```python
from build123d import *

# Parameters (mm, degrees)
EXTRUDE_1_DEPTH          = 4
SKETCH_3_R               = 4.330127019
SKETCH_3_R_2             = 2
EXTRUDE_2_DEPTH          = 9
SKETCH_4_R               = 1.5
CUT_EXTRUDE_1_DEPTH      = 15
CUT_EXTRUDE_2_DEPTH      = 15.585952146
CUT_EXTRUDE_2_DEPTH_BACK = 15.585952146
SKETCH_5_R               = 1.5


with BuildPart() as part:
    # 草图2 → 凸台-拉伸1 (new body)
    with BuildSketch(Plane(origin=(0, 0, 0), x_dir=(1, 0, 0), z_dir=(0, 1, 0))):
        Polygon((0, 0), (-2.5, 4.330127019), (-5, 0), align=None)
        Polygon((-2.5, -4.330127019), (-5, 0), (0, 0), align=None)
        Polygon((0, 0), (-2.5, -4.330127019), (2.5, -4.330127019), align=None)
        Polygon((0, 0), (2.5, -4.330127019), (5, 0), align=None)
        Polygon((0, 0), (5, 0), (2.5, 4.330127019), align=None)
        Polygon((0, 0), (2.5, 4.330127019), (-2.5, 4.330127019), align=None)
    extrude(amount=EXTRUDE_1_DEPTH)

    # 草图3 → 凸台-拉伸2 (add)
    with BuildSketch(Plane(origin=(0, 4, 0), x_dir=(1, 0, 0), z_dir=(0, 1, 0))):
        with Locations(Location((0, 0, 0), (0, 0, 270))):
            Circle(SKETCH_3_R)
        with Locations(Location((0, 0, 0), (0, 0, 270))):
            Circle(SKETCH_3_R_2, mode=Mode.SUBTRACT)
    extrude(amount=EXTRUDE_2_DEPTH)

    # 草图4 → 切除-拉伸1 (cut)
    with BuildSketch(Plane.XZ):
        with Locations(Location((0, 0, 0), (0, 0, 270))):
            Circle(SKETCH_4_R)
    extrude(amount=-CUT_EXTRUDE_1_DEPTH, mode=Mode.SUBTRACT)

    # 草图5 → 切除-拉伸2 (cut, two sides: drawn at the far end of the back side and taken through both)
    with BuildSketch(Plane(origin=(0, 0, 0), x_dir=(0, 0, -1), z_dir=(1, 0, 0)).offset(-CUT_EXTRUDE_2_DEPTH_BACK)):
        with Locations((0, 8)):
            Circle(SKETCH_5_R)
    extrude(amount=CUT_EXTRUDE_2_DEPTH + CUT_EXTRUDE_2_DEPTH_BACK, mode=Mode.SUBTRACT)


solid = part.part
```
Here's how the part is built. I have some questions about the finished solid (model axes, mm). A direction names the side the tool comes from. Round coordinates to 2 decimals unless told otherwise and drop trailing zeros. Order: outer loops, then holes, each group sorted by start corner. A loop starts at its lowest first (then second) coordinate and runs counter-clockwise, first axis right, second up. Notation, with made-up numbers: (52, 35.25) -> (96, 35.25) arc R18 cw to (96, 67.25) -> close; hole circle Ø7 at (-3, 85). An arc over 180 degrees is marked (long way). Use a Markdown table: item, result. Add a question column.
(1) If we mould it in two halves opening along Z, with no side actions, what happens to faces 1 (the face through (-3.73, 1.97, 2.2)), 2 (the face through (-2.848, 9.265, -0.806)), 3 (the face through (1.3, 8.44, 4.13))? For each: released by +Z, released by -Z, zero draft, split by the parting line, or undercut.
(2) For pin 1 Ø3 at (x, z) = (0.5, 0.5) entering from +Y; pin 2 Ø4 at (y, z) = (2, 0.5) entering from +X; pin 3 Ø3.5 at (x, z) = (0, 0) entering from +Y; pin 4 Ø2 at (y, z) = (4, 1.5) entering from -X, each with a flat end and sliding along its axis, tell me the tip position at first contact or that it passes through.
(3) For faces 4 (the face through (-2.3, 4, -3.9)), 5 (the face through (4.5, 4, 0)), 6 (the face through (2.3, 4, 3.9)), which set-ups out of +Z, -Z, +X, -X, +Y, -Y let a thin tool reach every point of the face, with its end or its side?
(4) Suppose I cut it at C-C, the plane y = 8. Please give me the cut outline in (x, z), and give its area (3 significant figures).
(5) Suppose I cut it at A-A, the plane y = 1. Please give me the cut outline in (x, z).
(6) I need wall thicknesses on line 1 along Y through (x, z) = (-2.15, 0); line 2 along Y through (x, z) = (-2.75, 3.75); line 3 along Z through (x, y) = (-1, 5). Which ranges of each line are inside material? Lowest first, please.
Verdict:
| question | item | result |
|---|---|---|
| 1 | face 1 | released by +Z |
| 1 | face 2 | undercut |
| 1 | face 3 | split by the parting line |
| 2 | pin 1 | y = 13 |
| 2 | pin 2 | x = 5 |
| 2 | pin 3 | y = 4 |
| 2 | pin 4 | x = -4.71 |
| 3 | face 4 | -Z, -X, +Y |
| 3 | face 5 | +X, +Y |
| 3 | face 6 | +Z, +X, +Y |
| 4 | outline | (-4.06, -1.5) arc R4.33 ccw to (4.06, -1.5) -> (1.32, -1.5) arc R2 cw to (-1.32, -1.5) -> close; (-4.06, 1.5) -> (-1.32, 1.5) arc R2 cw to (1.32, 1.5) -> (4.06, 1.5) arc R4.33 ccw to start |
| 4 | area | 31.6 mm2 |
| 5 | outline | (-5, 0) -> (-2.5, -4.33) -> (2.5, -4.33) -> (5, 0) -> (2.5, 4.33) -> (-2.5, 4.33) -> close; hole circle Ø3 at (0, 0) |
| 6 | line 1 | 0 to 6.5, 9.5 to 13 |
| 6 | line 2 | 0 to 4 |
| 6 | line 3 | -4.21 to -1.73, 1.73 to 4.21 |
